Design review of the part shown in the three views and the two pictorial views. Dimensions are in mm from the part's minimum x, y and z. Give positions to 0.01 mm unless a question says otherwise; leave off trailing zeros. Order: outer loops, then holes, each group sorted by start corner. A loop starts at its lowest first (then second) coordinate and runs counter-clockwise, first axis right, second up. Notation, with made-up numbers: M 25.25,72.5 L 77.25,72.5 A4 ccw 77.25,78.5 Z; hole C 27,81.5 d10. An arc over 180 degrees is marked long. Answer as a JSON object with one key per item and string values.
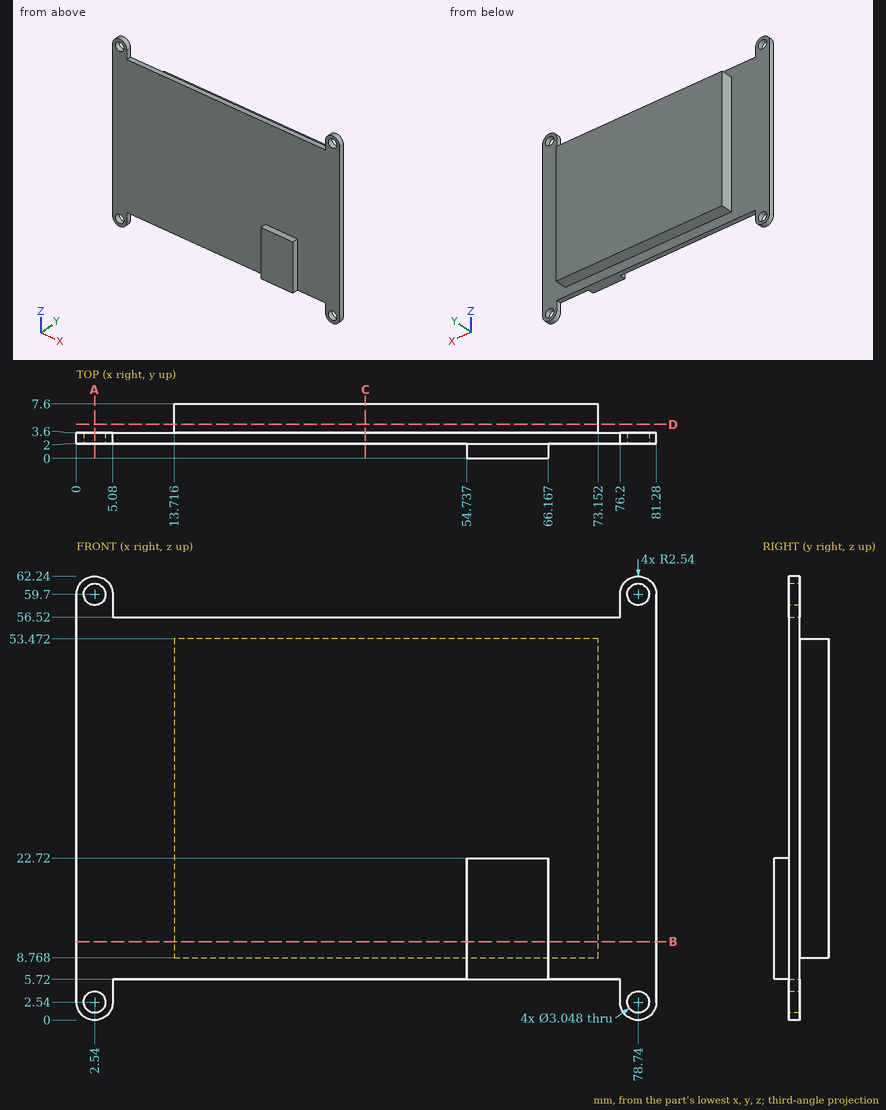
(1) We need section B-B (z = 11). Write out the cut boundary in (x, y), plus the area to 3 significant figures.
Checked values:
{"outline": "M 0,2 L 54.74,2 L 54.74,0 L 66.17,0 L 66.17,2 L 81.28,2 L 81.28,3.6 L 73.15,3.6 L 73.15,7.6 L 13.72,7.6 L 13.72,3.6 L 0,3.6 Z", "area": "391 mm^2"}
(2) We need section C-C (x = 40.5). Write out the cut boundary in (y, z), plus the area to 3 significant figures.
Checked values:
{"outline": "M 2,5.72 L 3.6,5.72 L 3.6,8.77 L 7.6,8.77 L 7.6,53.47 L 3.6,53.47 L 3.6,56.52 L 2,56.52 Z", "area": "260 mm^2"}
(3) We need section A-A (x = 2.54). Write out the cut boundary in (y, z), plus the area to 3 significant figures.
Checked values:
{"outline": "M 2,0 L 3.6,0 L 3.6,1.02 L 2,1.02 Z; M 2,4.06 L 3.6,4.06 L 3.6,58.18 L 2,58.18 Z; M 2,61.22 L 3.6,61.22 L 3.6,62.24 L 2,62.24 Z", "area": "89.8 mm^2"}
(4) To check wall thickness, follow L1, parallel to X at y = 3.1, z = 59.7; L2, parallel to X at y = 7.25, z = 34; L3, parallel to Y at x = 23.5, z = 19.5. State the ranges of each line that lie inside material, in increasing order. Write a range as from..to.
Checked values:
{"L1": "x = 0..1.02, 4.06..5.08, 76.2..77.22, 80.26..81.28", "L2": "x = 13.72..73.15", "L3": "y = 2..7.6"}
(5) We need section D-D (y = 4.75). Write out the cut boundary in (x, z), plus the area to 3 significant figures.
Checked values:
{"outline": "M 13.72,8.77 L 73.15,8.77 L 73.15,53.47 L 13.72,53.47 Z", "area": "2,660 mm^2"}
(6) Insertion check: pin 1 (4 mm diameter, centred on x = 45.5, y = 2.5, fed in from -Z); pin 2 (1 mm diameter, centred on x = 61.5, y = 1, fed in from +Z); pin 3 (3 mm diameter, centred on y = 5.5, z = 33, fed in from -X). Each pin has a flat end and moves straight along its axis. Give the tip position at first contact, or say it passes through.
Checked values:
{"pin 1": "stops at z = 5.72", "pin 2": "stops at z = 22.72", "pin 3": "stops at x = 13.72"}
